Work out the finished part from the listing and answer in its coordinate system (mm). Coordinates: 2 decimals unless noted, no trailing zeros. Order: outer loops, then holes, each group sorted by start corner. A loop starts at its lowest first (then second) coordinate and runs counter-clockwise, first axis right, second up. Notation, with made-up numbers: (-12.5, 59) - (33.5, 59) arc R31 cw to (33.5, 90) - close; hole circle Ø10 at (-19, 47.5). An arc over 180 degrees is marked (long way). Answer as a JSON object with one key per item and string values. Group by question number.
1) Find the intervals of material crossed by line 1 along Y through (x, z) = (0, 0.7) (3 decimals); line 2 along Y through (x, z) = (-39, 0.3); line 3 along Y through (x, z) = (25.5, 2.4), in increasing order.
2) Section C-C (x = -22) is taken. Give the vertices of the cut face in (y, z), plus the area to 3 significant figures.
3) Section A-A (x = 0) is taken. Give the vertices of the cut face in (y, z) (3 decimals).
4) Section D-D (y = -23) is taken. Give the vertices of the cut face in (x, z).
5) Each of these flat-tipped pins is pushed along its axis until it touches: P1, Ø1.4, axis at y = -1, z = 1, coming from the +X side; P2, Ø1.5, axis at y = 35, z = 0.5, coming from the +X side; P3, Ø1.4, axis at x = -37.5, z = 2, coming from the +Y side; P4, Ø2, axis at x = -33.5, y = 24, coming from the -Z side. Where does it stop, or does it pass through?
from build123d import *

# Parameters (mm, degrees)
F0_R     = 44.45
F0_W     = 5.207
F0_H     = 10.414
F0_W_2   = 10.414
F0_H_2   = 5.207
F0_R_2   = 19.685
F1_DEPTH = 2.794


with BuildPart() as f1:
    # F0 (on Top) → F1 (new body)
    with BuildSketch(Plane.XY):
        Circle(F0_R)
        Polygon((-24.20179, -20.519885), (-20.519885, -24.20179), (-27.883695, -31.5656), (-31.5656, -27.883695), align=None, mode=Mode.SUBTRACT)
        Polygon((-14.506919, -28.219526), (-9.696278, -30.212159), (-13.681543, -39.83344), (-18.492184, -37.840808), align=None, mode=Mode.SUBTRACT)
        Polygon((-30.212159, -9.696278), (-28.219526, -14.506919), (-37.840808, -18.492184), (-39.83344, -13.681543), align=None, mode=Mode.SUBTRACT)
        with Locations((0, -36.83)):
            Rectangle(F0_W, F0_H, mode=Mode.SUBTRACT)
        Polygon((9.696278, -30.212159), (14.506919, -28.219526), (18.492184, -37.840808), (13.681543, -39.83344), align=None, mode=Mode.SUBTRACT)
        Polygon((20.519885, -24.20179), (24.20179, -20.519885), (31.5656, -27.883695), (27.883695, -31.5656), align=None, mode=Mode.SUBTRACT)
        Polygon((28.219526, -14.506919), (30.212159, -9.696278), (39.83344, -13.681543), (37.840808, -18.492184), align=None, mode=Mode.SUBTRACT)
        with Locations((-36.83, 0)):
            Rectangle(F0_W_2, F0_H_2, mode=Mode.SUBTRACT)
        Polygon((-28.219526, 14.506919), (-30.212159, 9.696278), (-39.83344, 13.681543), (-37.840808, 18.492184), align=None, mode=Mode.SUBTRACT)
        Polygon((-20.519885, 24.20179), (-24.20179, 20.519885), (-31.5656, 27.883695), (-27.883695, 31.5656), align=None, mode=Mode.SUBTRACT)
        Polygon((-9.696278, 30.212159), (-14.506919, 28.219526), (-18.492184, 37.840808), (-13.681543, 39.83344), align=None, mode=Mode.SUBTRACT)
        Circle(F0_R_2, mode=Mode.SUBTRACT)
        with Locations((36.83, 0)):
            Rectangle(F0_W_2, F0_H_2, mode=Mode.SUBTRACT)
        Polygon((30.212159, 9.696278), (28.219526, 14.506919), (37.840808, 18.492184), (39.83344, 13.681543), align=None, mode=Mode.SUBTRACT)
        with Locations((0, 36.83)):
            Rectangle(F0_W, F0_H, mode=Mode.SUBTRACT)
        Polygon((14.506919, 28.219526), (9.696278, 30.212159), (13.681543, 39.83344), (18.492184, 37.840808), align=None, mode=Mode.SUBTRACT)
        Polygon((24.20179, 20.519885), (20.519885, 24.20179), (27.883695, 31.5656), (31.5656, 27.883695), align=None, mode=Mode.SUBTRACT)
    extrude(amount=F1_DEPTH)


solid = f1.part
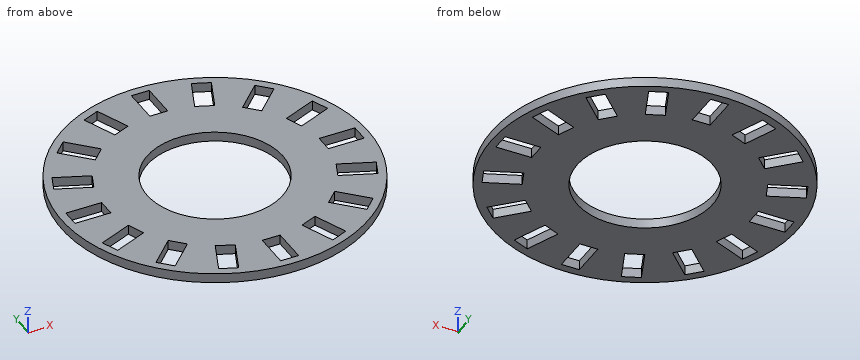
Report:
{
 "1": {"line 1": "y = -44.45 to -42.037, -31.623 to -19.685, 19.685 to 31.623, 42.037 to 44.45", "line 2": "y = -21.33 to -15.69, -13.34 to -2.6, 2.6 to 13.34, 15.69 to 21.33", "line 3": "y = -36.41 to -29.18, -21.82 to 21.82, 29.18 to 36.41"},
 "2": {"outline": "(-38.62, 0) - (-25.68, 0) - (-25.68, 2.79) - (-38.62, 2.79) - close; (-22.72, 0) - (22.72, 0) - (22.72, 2.79) - (-22.72, 2.79) - close; (25.68, 0) - (38.62, 0) - (38.62, 2.79) - (25.68, 2.79) - close", "area": "199 mm²"},
 "3": {"outline": "(-44.45, 0) - (-42.037, 0) - (-42.037, 2.794) - (-44.45, 2.794) - close; (-31.623, 0) - (-19.685, 0) - (-19.685, 2.794) - (-31.623, 2.794) - close; (19.685, 0) - (31.623, 0) - (31.623, 2.794) - (19.685, 2.794) - close; (42.037, 0) - (44.45, 0) - (44.45, 2.794) - (42.037, 2.794) - close"},
 "4": {"outline": "(-38.04, 0) - (-26.68, 0) - (-26.68, 2.79) - (-38.04, 2.79) - close; (-21.72, 0) - (21.72, 0) - (21.72, 2.79) - (-21.72, 2.79) - close; (26.68, 0) - (38.04, 0) - (38.04, 2.79) - (26.68, 2.79) - close"},
 "5": {"P1": "stops at x = 44.45", "P2": "stops at x = 28.33", "P3": "stops at y = 24.93", "P4": "stops at z = 0"}
}
